The model under review builds one solid part; all positions refer to its coordinate system, in mm. A direction names the side the tool comes from. Round coordinates to 2 decimals unless told otherwise and drop trailing zeros. Loops run counter-clockwise (first coordinate to the right, second up) from the corner with the lowest first, then second, coordinate; pieces in that order, holes last. Notation, with made-up numbers: (18, -25.75) -> (38, -25.75) arc R11 ccw to (38, -9.75) -> close; hole circle Ø1 at (-28.75, 77.25). An arc over 180 degrees is marked (long way). Use a Markdown table: item, result. Add a question column.
1) Insertion check: pin 1 (4 mm diameter, centred on y = -1, z = -3, fed in from +X); pin 2 (1.5 mm diameter, centred on y = -1, z = -2, fed in from -X); pin 3 (6.5 mm diameter, centred on y = -1, z = 4, fed in from +X); pin 4 (8 mm diameter, centred on x = 1.5, y = -4, fed in from -Z). Each pin has a flat end and moves straight along its axis. Give the tip position at first contact, or say it passes through.
2) Wall thickness on probe 1 along Y at (x, z) = (3.25, 5.5); probe 2 along X at (y, z) = (-1.75, -2.5); probe 3 along Z at (x, y) = (-11, 5.75): over which ranges is each line inside the solid? List them lowest first.
3) Mouldability with a two-part tool opening along Z and no side actions: class faces 5 (the cylindrical face through (-13.46, -0.08, -4.45)), 6 (the flat face through (12, -2.54, -2)), 7 (the cylindrical face through (12.2, -1.8, -5.6)) as released by +Z, released by -Z, zero draft, split by the parting line, or undercut.
4) Consider section C-C on z = -5.08. Give the boundary of the cut face in (x, y) (3 decimals), plus the area to 3 significant figures.
5) Consider section B-B on y = -3. Give the boundary of the cut face in (x, z).
6) For faces 1 (the cylindrical face through (-11.43, -0.15, 5.63)), 2 (the cylindrical face through (13.46, -0.08, -4.45)), 3 (the flat face through (-12, 2.54, -2)), 4 (the flat face through (11.43, 0, -3)), list the 3-axis set-ups (+Z, -Z, +X, -X, +Y, -Y) from which the entire face can be reached by the end or side of a thin tool; tool diameter is ignored.
7) Consider section A-A on x = -3. Give the boundary of the cut face in (y, z).
from build123d import *

# Parameters (mm, degrees)
F1_DEPTH  = 22.86
F3_DEPTH  = 6.35
F4_R      = 0.635
F5_DEPTH  = 1.5691231
F6_R      = 2.53999
F7_R      = 0.635
F9_DEPTH  = 6.35
F11_D     = 2.54
F16_D     = 127
F16_DEPTH = 17.781


# Not quite as in the source:
# - a fillet or chamfer is up to 0.001 mm smaller than in the source, because OpenCascade refuses the exact size
# - a length typed as a fraction of an inch, garbled in the dataset ("3 / 203.2 mm" for 3/8 in), is restored
# - the program builds the solid bodies; features that only make, move or delete a surface that nothing else refers to are left out


with BuildPart() as f1:
    # F0 (on Top) → F1 (new body)
    with BuildSketch(Plane.XY):
        Polygon((6.6501818182, 11.43), (0, 11.43), (-6.6501818182, 11.43), (-13.9976640991, 4.0825177191), (-13.9976640991, 0), (-13.9976640991, -4.0825177191), (-6.6501818182, -11.43), (0, -11.43), (6.6501818182, -11.43), (13.9976640991, -4.0825177191), (13.9976640991, 0), (13.9976640991, 4.0825177191), align=None)
        with BuildLine():
            ThreePointArc((6.5717879374, 9.3518181818), (10.1429886159, 5.26922024), (11.43, 0))
            ThreePointArc((11.43, 0), (10.1429886159, -5.26922024), (6.5717879374, -9.3518181818))
            Line((6.5717879374, -9.3518181818), (0, -9.3518181818))
            Line((0, -9.3518181818), (-6.5717879374, -9.3518181818))
            ThreePointArc((-6.5717879374, -9.3518181818), (-10.1429886159, -5.26922024), (-11.43, 0))
            ThreePointArc((-11.43, 0), (-10.1429886159, 5.26922024), (-6.5717879374, 9.3518181818))
            Line((-6.5717879374, 9.3518181818), (0, 9.3518181818))
            Line((0, 9.3518181818), (6.5717879374, 9.3518181818))
        make_face(mode=Mode.SUBTRACT)
    extrude(amount=F1_DEPTH)

    # F2 (on Top) → F3 (join)
    with BuildSketch(Plane.XY):
        Polygon((12.9991231, -2.54), (12.9991231, 0), (12.9991231, 2.54), (11.43, 2.54), (11.43, 0), (11.43, -2.54), align=None)
    extrude(amount=-F3_DEPTH)

    # F4 (on face) → F5 (join)
    with BuildSketch(Plane.YZ.offset(12.9991231)):
        with Locations((0, -5.08)):
            Circle(F4_R)
    extrude(amount=F5_DEPTH)

    # F6 (radius 2.54 in the source; OpenCascade refuses exactly that, so slightly less here)
    f6_edges = [f1.edges().sort_by_distance(p)[0] for p in [
        (12.214562, -2.54, -6.35),
        (12.214562, 2.54, -6.35),
    ]]
    fillet(f6_edges, radius=F6_R)

    # F7
    f7_edges = [f1.edges().sort_by_distance(p)[0] for p in [
        (14.568246, -0.635, -5.08),
    ]]
    fillet(f7_edges, radius=F7_R)

    # F8 (on face) → F9 (join)
    with BuildSketch(Plane.XY.offset(22.86)):
        Polygon((13.9976640991, 2.54), (12.4285360385, 2.54), (12.4285360385, 0), (12.4285360385, -2.54), (13.9976640991, -2.54), (13.9976640991, 0), align=None)
    extrude(amount=F9_DEPTH)

    # F11 (through all)
    with Locations(Plane.YZ.offset(13.9976640991)):
        with Locations((0, 26.67)):
            Hole(F11_D / 2)

    # F12: F1 across plane


with BuildPart() as f1_1:
    add(f1.part)
    add(f1.part.mirror(Plane.YZ))

    # F16 (through all, one way)
    with BuildSketch(Plane(origin=(0, 0, 11.43), x_dir=(1, 0, 0), z_dir=(0, 0, -1))):
        with Locations((0, 0)):
            Circle(F16_D / 2)
    extrude(amount=-F16_DEPTH, mode=Mode.SUBTRACT)


solid = f1_1.part
Result set:
| question | item | result |
|---|---|---|
| 1 | pin 1 | x = 14.49 |
| 1 | pin 2 | x = -13 |
| 1 | pin 3 | x = 14 |
| 1 | pin 4 | through |
| 2 | probe 1 | -11.43 to -9.35, 9.35 to 11.43 |
| 2 | probe 2 | -13 to -11.43, 11.43 to 13 |
| 2 | probe 3 | 0 to 11.43 |
| 3 | face 5 | undercut |
| 3 | face 6 | zero draft |
| 3 | face 7 | released by -Z |
| 4 | outline | (-13.933, -0.635) -> (-12.999, -0.635) -> (-12.999, -2.2) -> (-11.43, -2.2) -> (-11.43, 2.2) -> (-12.999, 2.2) -> (-12.999, 0.635) -> (-13.933, 0.635) arc R0.635 ccw to start; (11.43, -2.2) -> (12.999, -2.2) -> (12.999, -0.635) -> (13.933, -0.635) arc R0.635 ccw to (13.933, 0.635) -> (12.999, 0.635) -> (12.999, 2.2) -> (11.43, 2.2) -> close |
| 4 | area | 17.4 mm2 |
| 5 | outline | (-14, 0) -> (-11.03, 0) -> (-11.03, 11.43) -> (-14, 11.43) -> close; (11.03, 0) -> (14, 0) -> (14, 11.43) -> (11.03, 11.43) -> close |
| 6 | face 1 | +Z, -Z |
| 6 | face 2 | +X |
| 6 | face 3 | -Z, +X, -X, +Y |
| 6 | face 4 | -Z, +Y, -Y |
| 7 | outline | (-11.43, 0) -> (-9.35, 0) -> (-9.35, 11.43) -> (-11.43, 11.43) -> close; (9.35, 0) -> (11.43, 0) -> (11.43, 11.43) -> (9.35, 11.43) -> close |
